Here's how the part is built. I have some questions about the finished solid (model axes, mm). Coordinates: 2 decimals unless noted, no trailing zeros. Loops run counter-clockwise (first coordinate to the right, second up) from the corner with the lowest first, then second, coordinate; pieces in that order, holes last. Notation, with made-up numbers: (-4.5, -6) - (8.5, -6) arc R20 ccw to (8.5, 29) - close; hole circle Ø8 at (69.25, 75.25). An arc over 180 degrees is marked (long way). Use a Markdown table: item, result.
```python
from build123d import *


with BuildPart() as f1:
    # F0 (on Front) → F1 (revolve)
    with BuildSketch(Plane.XZ):
        with BuildLine():
            Line((105.4, 0), (106.4, 0))
            ThreePointArc((106.4, 0), (107.5682, 2.693302), (104.803506, 1.705864))
            ThreePointArc((104.803506, 1.705864), (98.126839, 2.584605), (91.808444, 4.914402))
            ThreePointArc((91.808444, 4.914402), (57.62064, 31.81586), (36.776793, 70))
            Line((36.776793, 70), (35, 70))
            ThreePointArc((35, 70), (56.154601, 30.917261), (91.046937, 3.394498))
            ThreePointArc((91.046937, 3.394498), (98.025499, 0.86017), (105.4, 0))
        make_face()
    revolve(axis=Axis((0, 0, 35), (0, 0, 1)))


solid = f1.part
```
Q1. I want a section at B-B, the plane z = 37. Write out the boundary of the cut face in (x, y).
Check values:
| item | result |
|---|---|
| outline | circle Ø107 at (0, 0); hole circle Ø102.78 at (0, 0) |
Q2. Will these pins go through, and if not, where does the flat tip stop? P1, Ø3, axis at x = -69.5, y = -13.5, coming from the -Z side; P2, Ø8, axis at x = 16.5, z = 35, coming from the -Y side; P3, Ø1.5, axis at y = 17.5, z = 31, coming from the +X side.
Check values:
| item | result |
|---|---|
| P1 | z = 15.3 |
| P2 | y = -56.11 |
| P3 | x = 56.35 |
Q3. Please list where these lines run through material, in increasing order: L1, parallel to X at y = 32, z = 43.5; L2, parallel to X at y = -31.5, z = 18.5; L3, parallel to Z at x = -56.5, y = 90. Write a range as from..to.
Check values:
| item | result |
|---|---|
| L1 | -37.13..-34.43, 34.43..37.13 |
| L2 | -63.67..-60.73, 60.73..63.67 |
| L3 | 0..3.19 |
Q4. I want a section at A-A, the plane z = 25. Write out the boundary of the cut face in (x, y), then the cut area to 3 significant figures.
Check values:
| item | result |
|---|---|
| outline | circle Ø127.81 at (0, 0); hole circle Ø123.02 at (0, 0) |
| area | 942 mm^2 |
